Build history of the part. All positions in model axes, mm. A direction names the side the tool comes from. Give positions to 0.01 mm unless a question says otherwise; leave off trailing zeros. Order: outer loops, then holes, each group sorted by start corner. A loop starts at its lowest first (then second) coordinate and runs counter-clockwise, first axis right, second up. Notation, with made-up numbers: M 6,88 L 14,88 A9 cw 14,103 Z; hole C 68,-37 d8. An arc over 180 degrees is marked long. One line per item, written item: value. Start each with the question number.
from build123d import *

# Parameters (mm, degrees)
F4_DEPTH      = 305.001
F4_DEPTH_BACK = 305.001
F6_D          = 9
F6_DEPTH      = 305.001
F8_D          = 9


with BuildPart() as f2:
    # F2: sweep along a path in F0
    with BuildLine(Plane.XY) as f2_path:
        Line((305, 0), (305, 75))
        Line((305, 75), (90, 800))
        Line((90, 800), (0, 800))
        Line((0, 800), (-90, 800))
        Line((-90, 800), (-305, 75))
        Line((-305, 75), (-305, 0))
    # F1 (on Front) → F2 (sweep)
    with BuildSketch(Plane.XZ):
        Polygon((265, 0), (305, 0), (305, 40), (302, 40), (302, 3), (265, 3), align=None)
    sweep(path=f2_path.line, transition=Transition.RIGHT)

    # F3 (on Right) → F4 (cut, two sides)
    with BuildSketch(Plane.YZ) as f4_sk:
        with BuildLine():
            ThreePointArc((15, 0), (4.1666666667, 7.5), (0, 20))
            Line((0, 20), (0, 0))
            Line((0, 0), (15, 0))
        make_face()
        with BuildLine():
            ThreePointArc((0, 20), (4.1666666667, 32.5), (15, 40))
            Line((15, 40), (0, 40))
            Line((0, 40), (0, 20))
        make_face()
    extrude(amount=-F4_DEPTH, mode=Mode.SUBTRACT)
    extrude(f4_sk.sketch, amount=F4_DEPTH_BACK, mode=Mode.SUBTRACT)

    # F6 (through all, one way)
    with BuildSketch(Plane.YZ):
        with Locations((20.8333333333, 20)):
            Circle(F6_D / 2)
    extrude(amount=-F6_DEPTH, mode=Mode.SUBTRACT)

    # F8 (through all)
    with Locations(Plane(origin=(0, 0, 0), x_dir=(0, 1, 0), z_dir=(-1, 0, 0))):
        with Locations((20.8333333333, -20)):
            Hole(F8_D / 2)


solid = f2.part
1) Drill centre lines: line 1 (X direction, y = 52.5, z = 25); line 2 (X direction, y = 129, z = 10); line 3 (Y direction, x = -56, z = 35). Where is each one in solid material? Low to high.
2) Slice it at D-D (x = 160.5). List the corners of the cut face in (y, z), plus the area to 3 significant figures.
3) Slice it at B-B (x = -32.5). List the corners of the cut face in (y, z).
4) Drop flat-ended pins along their axis: P1, Ø3, axis at y = 504, z = 25.5, coming from the -X side; P2, Ø3, axis at y = 698, z = 8, coming from the -X side; P3, Ø5, axis at y = 613, z = 31, coming from the +X side; P4, Ø5.5, axis at y = 20.83, z = 20, coming from the +X side. Give the stop position or say it passes through.
5) Pull direction X, two halves, no side cores. Call faces 4 (the flat face through (-305, 37, 20)), 5 (the flat face through (195.995, 442.575, 19.72)), 6 (the flat face through (158, 434, 3)): pulls with the +X half, pulls with the -X half, needs draft (parallel to the pull), parting line crosses it, or undercut.
6) Tool access for faces 1 (the flat face through (-164.004, 409.761, 1.521)), 2 (the flat face through (305, 38, 20)), 3 (the flat face through (-1, 797, 22)): list every direction of +Z, -Z, +X, -X, +Y, -Y with a clear straight run to the whole face (end or side of a thin tool).
7) Slice it at C-C (z = 33). List the corners of the cut face in (x, y).
8) Slice it at A-A (y = 190.5). List the corners of the cut face in (x, z).
Results list:
1. line 1: x = -305 to -302, 302 to 305
1. line 2: x = -288.99 to -285.86, 285.86 to 288.99
1. line 3: y = 797 to 800
2. outline: M 421.58,0 L 562.27,0 L 562.27,40 L 551.72,40 L 551.72,3 L 421.58,3 Z
2. area: 812 mm²
3. outline: M 760,0 L 800,0 L 800,40 L 797,40 L 797,3 L 760,3 Z
4. P1: stops at x = -178.22
4. P2: stops at x = -120.69
4. P3: stops at x = 146.2
4. P4: passes through
5. face 4: pulls with the -X half
5. face 5: pulls with the +X half
5. face 6: undercut
6. face 1: +Z, -Z, -Y
6. face 2: +Z, -Z, +X, +Y, -Y
6. face 3: +Z, -Y
7. outline: M -305,4.55 L -302,4.55 L -302,74.56 L -87.76,797 L 87.76,797 L 302,74.56 L 302,4.55 L 305,4.55 L 305,75 L 90,800 L -90,800 L -305,75 Z
8. outline: M -270.75,0 L -229.03,0 L -229.03,3 L -267.62,3 L -267.62,40 L -270.75,40 Z; M 229.03,0 L 270.75,0 L 270.75,40 L 267.62,40 L 267.62,3 L 229.03,3 Z
